from build123d import *

# Parameters (mm, degrees)
SKETCH1_R           = 3.175
SKETCH1_R_2         = 4.7625
BOSS_EXTRUDE1_DEPTH = 0.79375


with BuildPart() as part:
    # Sketch1 → Boss-Extrude1 (new body)
    with BuildSketch(Plane(origin=(0, 0, 0), x_dir=(1, 0, 0), z_dir=(0, 1, 0))):
        with BuildLine():
            Line((-81.75625, 112.7125), (81.75625, 112.7125))
            ThreePointArc((81.75625, 112.7125), (87.368910076, 110.387660076), (89.69375, 104.775))
            Line((89.69375, 104.775), (89.69375, -87.3125))
            ThreePointArc((89.69375, -87.3125), (82.254262242, -105.273012242), (64.29375, -112.7125))
            Line((64.29375, -112.7125), (-64.29375, -112.7125))
            ThreePointArc((-64.29375, -112.7125), (-82.254262242, -105.273012242), (-89.69375, -87.3125))
            Line((-89.69375, -87.3125), (-89.69375, 104.775))
            ThreePointArc((-89.69375, 104.775), (-87.368910076, 110.387660076), (-81.75625, 112.7125))
        make_face()
        with Locations(Location((-57.94375, 70.96125, 0), (0, 0, 270))):
            Circle(SKETCH1_R, mode=Mode.SUBTRACT)
        with Locations(Location((57.94375, 70.96125, 0), (0, 0, 270))):
            Circle(SKETCH1_R, mode=Mode.SUBTRACT)
        with Locations(Location((57.94375, -94.13875, 0), (0, 0, 270))):
            Circle(SKETCH1_R, mode=Mode.SUBTRACT)
        with Locations(Location((-57.94375, -94.13875, 0), (0, 0, 270))):
            Circle(SKETCH1_R, mode=Mode.SUBTRACT)
        with Locations(Location((-73.81875, -74.6125, 0), (0, 0, 270))):
            Circle(SKETCH1_R_2, mode=Mode.SUBTRACT)
        with Locations(Location((-73.81875, 77.7875, 0), (0, 0, 270))):
            Circle(SKETCH1_R_2, mode=Mode.SUBTRACT)
        with Locations(Location((73.81875, 77.7875, 0), (0, 0, 270))):
            Circle(SKETCH1_R_2, mode=Mode.SUBTRACT)
        with Locations(Location((73.81875, -74.6125, 0), (0, 0, 270))):
            Circle(SKETCH1_R_2, mode=Mode.SUBTRACT)
        with BuildLine():
            Line((-26.19375, -68.73748), (-13.49375, -68.73748))
            ThreePointArc((-13.49375, -68.73748), (-3.96875, -78.26248), (-13.49375, -87.78748))
            Line((-13.49375, -87.78748), (-26.19375, -87.78748))
            ThreePointArc((-26.19375, -87.78748), (-35.71875, -78.26248), (-26.19375, -68.73748))
        make_face(mode=Mode.SUBTRACT)
        with BuildLine():
            Line((26.19375, -68.73748), (13.49375, -68.73748))
            ThreePointArc((13.49375, -68.73748), (3.96875, -78.26248), (13.49375, -87.78748))
            Line((13.49375, -87.78748), (26.19375, -87.78748))
            ThreePointArc((26.19375, -87.78748), (35.71875, -78.26248), (26.19375, -68.73748))
        make_face(mode=Mode.SUBTRACT)
        with BuildLine():
            Line((-43.34637, 46.94682), (-43.34637, 3.85572))
            ThreePointArc((-43.34637, 3.85572), (-60.52947, -13.32738), (-77.71257, 3.85572))
            Line((-77.71257, 3.85572), (-77.71257, 46.94682))
            ThreePointArc((-77.71257, 46.94682), (-60.52947, 64.12992), (-43.34637, 46.94682))
        make_face(mode=Mode.SUBTRACT)
        with BuildLine():
            Line((43.34637, 46.94682), (43.34637, 3.85572))
            ThreePointArc((43.34637, 3.85572), (60.52947, -13.32738), (77.71257, 3.85572))
            Line((77.71257, 3.85572), (77.71257, 46.94682))
            ThreePointArc((77.71257, 46.94682), (60.52947, 64.12992), (43.34637, 46.94682))
        make_face(mode=Mode.SUBTRACT)
    extrude(amount=BOSS_EXTRUDE1_DEPTH)


solid = part.part
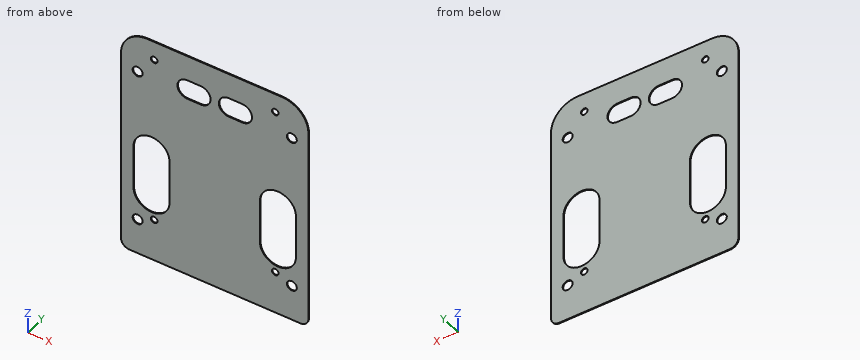
For this review, take the finished solid that the model builds, in its own axes (mm). Round coordinates to 2 decimals unless told otherwise and drop trailing zeros. Loops run counter-clockwise (first coordinate to the right, second up) from the corner with the lowest first, then second, coordinate; pieces in that order, holes last. Notation, with made-up numbers: (42, -23.75) - (77, -23.75) arc R17 cw to (77, 1.25) - close; hole circle Ø11 at (31, 31.25). An arc over 180 degrees is marked (long way). One line per item, written item: value. Start each with the question number.
Item 1: Take a section at D-D (x = -6.5). Give the boundary of the cut face in (y, z).
Item 2: Take a section at C-C (y = 0.35). State how many separate pieces and enclosed holes the cut face has, plus the area to 3 significant figures.
Item 3: Take a section at B-B (x = 18). Give the boundary of the cut face in (y, z), plus the area to 3 significant figures.
Item 4: Take a section at A-A (z = -11.5). Give the boundary of the cut face in (x, y).
Item 5: For L1, parallel to X at y = 0.15, z = -36.5; L2, parallel to Z at x = 71, y = 0.35; L3, parallel to X at y = 0.2, z = -56, list the stretches that pass through material, from the lowest coordinate up.
Answer below:
1. outline: (0, -112.71) - (0.79, -112.71) - (0.79, 71.8) - (0, 71.8) - close; (0, 84.73) - (0.79, 84.73) - (0.79, 112.71) - (0, 112.71) - close
2. separate pieces: 1
2. enclosed holes: 12
2. area: 33,900 mm2
3. outline: (0, -112.71) - (0.79, -112.71) - (0.79, 68.74) - (0, 68.74) - close; (0, 87.79) - (0.79, 87.79) - (0.79, 112.71) - (0, 112.71) - close
3. area: 164 mm2
4. outline: (-89.69, 0) - (-77.71, 0) - (-77.71, 0.79) - (-89.69, 0.79) - close; (-43.35, 0) - (43.35, 0) - (43.35, 0.79) - (-43.35, 0.79) - close; (77.71, 0) - (89.69, 0) - (89.69, 0.79) - (77.71, 0.79) - close
5. L1: x = -89.69 to -77.71, -43.35 to 43.35, 77.71 to 89.69
5. L2: z = -112.71 to -81.63, -73.95 to -60.57, 9.77 to 70.77, 78.45 to 111.81
5. L3: x = -89.69 to -75.13, -45.92 to 45.92, 75.13 to 89.69
